Geometry: final body of the model. Coordinates: model frame, mm. A direction names the side the tool comes from. Give positions to 0.01 mm unless a question says otherwise; leave off trailing zeros. Loops run counter-clockwise (first coordinate to the right, second up) from the corner with the lowest first, then second, coordinate; pieces in that order, holes last. Notation, with made-up numbers: (13.5, 0.5) -> (69.5, 0.5) arc R7 ccw to (69.5, 6.5) -> close; hole circle Ø1 at (-39, 12.5). An arc over 180 degrees is marked (long way). Answer in a Markdown table with one row per item. Add a question column.
from build123d import *

# Parameters (mm, degrees)
BOSS_EXTRUDE1_DEPTH     = 1
BOSS_EXTRUDE2_START     = 1
BOSS_EXTRUDE2_DEPTH     = 2
CUT_EXTRUDE1_DEPTH      = 29.565825694
CUT_EXTRUDE1_DEPTH_BACK = 30.565825694
CUT_EXTRUDE1_START      = 1
SKETCH1_4_W             = 10
SKETCH1_4_H             = 4
SKETCH1_4_W_2           = 2
SKETCH1_4_H_2           = 3
SKETCH1_4_W_3           = 3.497046445
SKETCH1_4_H_3           = 4.9
BOSS_EXTRUDE3_START     = -20.304052
SKETCH2_W               = 2.6
SKETCH2_H               = 1.1
BOSS_EXTRUDE3_DEPTH     = 0.6
BOSS_EXTRUDE4_START     = 20.195948
SKETCH2_2_W             = 2.6
SKETCH2_2_H             = 1.1
BOSS_EXTRUDE4_DEPTH     = 0.6


with BuildPart() as part:
    # Sketch1 → Boss-Extrude1 (new body)
    with BuildSketch(Plane(origin=(0, 0, 0), x_dir=(1, 0, 0), z_dir=(0, 1, 0))):
        Polygon((-20.304052055, 14.886180374), (-20.304052055, -14.649453395), (-15.437733663, -19.631636511), (15.329629553, -19.631636511), (20.195947945, -14.649453395), (20.195947945, 14.886180374), (15.329629553, 19.868363489), (-15.437733663, 19.868363489), align=None)
    extrude(amount=BOSS_EXTRUDE1_DEPTH)

    # Sketch1<3> → Boss-Extrude2 (add)
    with BuildSketch(Plane(origin=(0, 0, 0), x_dir=(1, 0, 0), z_dir=(0, 1, 0)).offset(BOSS_EXTRUDE2_START)):
        Polygon((-20.304052055, 14.886180374), (-20.304052055, -14.649453395), (-15.437733663, -19.631636511), (15.329629553, -19.631636511), (20.195947945, -14.649453395), (20.195947945, 14.886180374), (15.329629553, 19.868363489), (-15.437733663, 19.868363489), align=None)
        Polygon((-19.304052055, 14.478841428), (-15.016611903, 18.868363489), (14.908507792, 18.868363489), (19.195947945, 14.478841428), (19.195947945, -14.24211445), (14.908507792, -18.631636511), (-15.016611903, -18.631636511), (-19.304052055, -14.24211445), align=None, mode=Mode.SUBTRACT)
    extrude(amount=BOSS_EXTRUDE2_DEPTH)

    # Sketch1<4> → Cut-Extrude1 (cut, two sides: drawn at the far end of the back side and taken through both)
    with BuildSketch(Plane(origin=(0, 0, 0), x_dir=(1, 0, 0), z_dir=(0, 1, 0)).offset(CUT_EXTRUDE1_START - CUT_EXTRUDE1_DEPTH_BACK)):
        with Locations((10.329629553, 17.868363489)):
            Rectangle(SKETCH1_4_W, SKETCH1_4_H)
        with Locations((-8.511953553, -17.131636511)):
            Rectangle(SKETCH1_4_W_2, SKETCH1_4_H_2)
        with Locations((-16.010445854, -13.139778313)):
            Rectangle(SKETCH1_4_W_3, SKETCH1_4_H_3)
    extrude(amount=CUT_EXTRUDE1_DEPTH + CUT_EXTRUDE1_DEPTH_BACK, mode=Mode.SUBTRACT)

    # Sketch2 → Boss-Extrude3 (add)
    with BuildSketch(Plane(origin=(0, 0, 0), x_dir=(0, 0, -1), z_dir=(1, 0, 0)).offset(BOSS_EXTRUDE3_START)):
        with Locations((-11.251288132, 1.75)):
            Rectangle(SKETCH2_W, SKETCH2_H)
        with Locations((11.48801511, 1.75)):
            Rectangle(SKETCH2_W, SKETCH2_H)
    extrude(amount=-BOSS_EXTRUDE3_DEPTH)

    # Sketch2<2> → Boss-Extrude4 (add)
    with BuildSketch(Plane(origin=(0, 0, 0), x_dir=(0, 0, -1), z_dir=(1, 0, 0)).offset(BOSS_EXTRUDE4_START)):
        with Locations((-11.251288132, 1.75)):
            Rectangle(SKETCH2_2_W, SKETCH2_2_H)
        with Locations((11.48801511, 1.75)):
            Rectangle(SKETCH2_2_W, SKETCH2_2_H)
    extrude(amount=BOSS_EXTRUDE4_DEPTH)


solid = part.part
(1) Reachability of faces 1 (the flat face through (-16, 0.5, 10.69)), 2 (the flat face through (-17.1, 2, 16.5)), 3 (the flat face through (-20.904, 2, -11)) from +Z, -Z, +X, -X, +Y, -Y: full face, straight path, thin tool, end or side. Return the list, or none.
(2) Cut plane B-B on x = -7. Return the cut outline in (y, z), then the cut area to 3 significant figures.
(3) Cut plane A-A on z = 4.5. Return the cut outline in (x, y), then the cut area to 3 significant figures.
(4) Cut plane C-C on x = 14. Return the cut outline in (y, z), then the cut area to 3 significant figures.
(5) Material intervals for line 1 along Z through (x, y) = (-2, 1.6); line 2 along X through (y, z) = (1.15, 12.5); line 3 along X through (y, z) = (1.9, -12), sorted ascending. Write a range as from..to.
(6) Pin query (flat end, axial travel): pin 1 Ø2 at (x, z) = (-5.5, -10.5) entering from -Y; pin 2 Ø0.5 at (y, z) = (0.5, 17.5) entering from -X; pin 3 Ø11 at (x, z) = (-9.5, -7.5) entering from +Y; pin 4 Ø0.9 at (y, z) = (1, -17.5) entering from -X. Return the tip coordinate at first contact, or that it passes through.
(7) Draft query along Z for faces 4 (the flat face through (5.33, 0.8, -18.3)), 5 (the flat face through (-17.84, 1.48, -17.41)), 6 (the flat face through (-7.512, 0.5, 17.2)). Return one class per face: +Z half, -Z half, draft (parallel to the pull), parting line (faces both ways), or undercut.
Answer list:
| question | item | result |
|---|---|---|
| 1 | face 1 | +Y, -Y |
| 1 | face 2 | +Y |
| 1 | face 3 | +Z, -Z, -X, +Y, -Y |
| 2 | outline | (0, -19.87) -> (3, -19.87) -> (3, -18.87) -> (1, -18.87) -> (1, 18.63) -> (3, 18.63) -> (3, 19.63) -> (0, 19.63) -> close |
| 2 | area | 43.5 mm² |
| 3 | outline | (-20.3, 0) -> (20.2, 0) -> (20.2, 3) -> (19.2, 3) -> (19.2, 1) -> (-19.3, 1) -> (-19.3, 3) -> (-20.3, 3) -> close |
| 3 | area | 44.5 mm² |
| 4 | outline | (0, -15.87) -> (1, -15.87) -> (1, 18.63) -> (3, 18.63) -> (3, 19.63) -> (0, 19.63) -> close |
| 4 | area | 37.5 mm² |
| 5 | line 1 | z = -19.87..-18.87, 18.63..19.63 |
| 5 | line 2 | x = -20.3..-19.3, 19.2..20.2 |
| 5 | line 3 | x = -20.9..-19.3, 19.2..20.8 |
| 6 | pin 1 | stops at y = 0 |
| 6 | pin 2 | stops at x = -17.76 |
| 6 | pin 3 | stops at y = 1 |
| 6 | pin 4 | stops at x = -18.19 |
| 7 | face 4 | draft |
| 7 | face 5 | -Z half |
| 7 | face 6 | undercut |
